Source: CAD feature listing. Evaluate the final solid. Frame: model axes, mm. A direction names the side the tool comes from. Round coordinates to 2 decimals unless told otherwise and drop trailing zeros. Loops run counter-clockwise (first coordinate to the right, second up) from the corner with the lowest first, then second, coordinate; pieces in that order, holes last.
Item 1: Section query C-C on y = 34. Return loops of the section in (x, z), then the cut area to 3 significant figures.
Item 2: Section query A-A on x = 10.16. Return loops of the section in (y, z).
Item 3: First-contact query: P1, Ø3, axis at x = 21.5, z = 47.5, coming from the +Y side; P2, Ø2.5, axis at y = 35, z = 43.5, coming from the +X side. Flat tips, straight axial feed; report the tip coordinate or a pass-through.
Item 4: Section query B-B on z = 44.75. Return loops of the section in (x, y), then the cut area to 3 significant figures.
Item 5: Pull-direction query (X, two-part tool) for faces 1 (the flat face through (10, 31, 41.178)), 2 (the flat face through (25.4, 17, 43)), 3 (the flat face through (13, 5.207, 43)); classes: released by +X, released by -X, zero draft, split by the parting line, or undercut.
Item 6: Section query D-D on z = 36.75. Return loops of the section in (x, y).
Item 7: Access query for faces 4 (the flat face through (20, 26.797, 47)), 5 (the cylindrical face through (12.158, 31.025, 37.958)), 6 (the flat face through (13, 21, 34.828)), 7 (the flat face through (0, 21, 43)), 8 (the flat face through (15.24, 33, 43)). Directions: +Z, -Z, +X, -X, +Y, -Y. A direction counts if a zero-diameter tool reaches every point of the face in a straight line with its end or side. Return the directions, or none.
Item 8: Ray query, L1, parallel to Z at x = 20.32, y = 28.7; L2, parallel to Y at x = 10.16, z = 38; L3, parallel to X at y = 35, z = 37.25. Return the intervals inside material, ascending.
Autodesk Inventor part; units mm, degrees
ref_plane "YZ Plane" through (0, 0, 0) normal (1, 0, 0) x (0, 1, 0)
ref_plane "XZ Plane" through (0, 0, 0) normal (0, 1, 0) x (-1, 0, 0)
ref_plane "XY Plane" through (0, 0, 0) normal (0, 0, 1) x (1, 0, 0)
sketch "Sketch1" plane through (0, 0, 0) normal (1, 0, 0) x (0, 1, 0)
  line L0 (36.9572, 50.7029) -> (5.2072, 50.7029)
  line L1 (5.2072, 50.7029) -> (5.2072, 34.8279)
  line L2 (5.2072, 34.8279) -> (36.9572, 34.8279)
  line L3 (36.9572, 34.8279) -> (36.9572, 50.7029)
  point P0 (0, 0)
  dimension "d0" = 31.75
  dimension "d1" = 15.875
extrude "Extrusion1" add sketch "Sketch1" along normal blind 25.4
sketch "Sketch2" plane through (0, 36.9572, 50.7029) normal (0, 1, 0) x (1, 0, 0)
  line L0 (25.4, 0) -> (25.4, 15.875)
  line L1 (0, 0) -> (25.4, 0)
  line L2 (25.4, 15.875) -> (15.24, 15.875)
  line L3 (15.24, 15.875) -> (15.24, 0)
  line L4 (15.24, 0) -> (25.4, 0)
  line L5 (25.4, 0) -> (25.4, 15.875)
  point P0 (0, 50.7029)
  dimension "d4" = 10.16
extrude "Extrusion2" cut sketch "Sketch2" against normal blind 7.62
sketch "Sketch3" plane through (0, 29.3372, 50.7029) normal (0, 1, 0) x (1, 0, 0)
  line L0 (15.24, 0) -> (15.24, 15.875)
  line L1 (25.4, 0) -> (15.24, 0)
  line L2 (25.4, 15.875) -> (25.4, 0)
  line L3 (15.24, 15.875) -> (25.4, 15.875)
  circle A0 centre (20.32, 3.5522) radius 2
  point P0 (0, 50.7029)
  dimension "d7" = 4
  dimension "d8" = 5.08
  dimension "d9" = 3.5522
extrude "Extrusion3" cut sketch "Sketch3" against normal blind 2.54 contours A0
sketch "Sketch4" plane through (0, 5.2072, 34.8279) normal (0, 0, -1) x (-1, 0, 0)
  circle A0 centre (-10.16, 25.7302) radius 2
  point P0 (0, -5.2072)
extrude "Extrusion4" cut sketch "Sketch4" against normal blind 6.35
properties part number "Meal inside front"
Data:
1. outline: (0, 34.83) - (15.24, 34.83) - (15.24, 50.7) - (0, 50.7) - close
1. area: 242 mm2
2. outline: (5.21, 34.83) - (28.94, 34.83) - (28.94, 41.18) - (32.94, 41.18) - (32.94, 34.83) - (36.96, 34.83) - (36.96, 50.7) - (5.21, 50.7) - close
3. P1: stops at y = 29.34
3. P2: stops at x = 15.24
4. outline: (0, 5.21) - (25.4, 5.21) - (25.4, 29.34) - (15.24, 29.34) - (15.24, 36.96) - (0, 36.96) - close
4. area: 729 mm2
5. face 1: undercut
5. face 2: released by +X
5. face 3: zero draft
6. outline: (0, 5.21) - (25.4, 5.21) - (25.4, 29.34) - (15.24, 29.34) - (15.24, 36.96) - (0, 36.96) - close; hole circle Ø4 at (10.16, 30.94)
7. face 4: +Y
7. face 5: -Z
7. face 6: -Z, +X, -X, +Y, -Y
7. face 7: +Z, -Z, -X, +Y, -Y
7. face 8: +Z, -Z, +X, +Y
8. L1: z = 34.83 to 45.15, 49.15 to 50.7
8. L2: y = 5.21 to 28.94, 32.94 to 36.96
8. L3: x = 0 to 15.24
